Here's how the part is built. I have some questions about the finished solid (model axes, mm). Face numbers are marked on the shaded views. Give positions to 0.01 mm unless a question says otherwise; leave off trailing zeros. Order: outer loops, then holes, each group sorted by start corner. A loop starts at its lowest first (then second) coordinate and runs counter-clockwise, first axis right, second up. Notation, with made-up numbers: (49.25, 13) -> (63.25, 13) arc R20 cw to (63.25, 20) -> close; hole circle Ø2 at (35, 25.25). An arc over 180 degrees is marked (long way). Write each question's results on one line, items separated by ' | '. Start each with the question number.
Q1. I need wall thicknesses on line 1 along X through (y, z) = (0, 10.5); line 2 along X through (y, z) = (0, 24.5); line 3 along Z through (x, y) = (-1, 4). Which ranges of each line are inside material? Lowest first, please. Write a range as [from, to].
Q2. Thinking about a two-plate mould opening in Z: for the marked faces 1 and 2, which applies, pulls with the +Z half, pulls with the -Z half, needs draft (parallel to the pull), parting line crosses it, or undercut?
Q3. Imagine slicing it at C-C, the plane z = 27.75. Please give me the cut outline in (x, y).
Q4. I'm going to push a flat-ended pin straight in: pin 1 (1 mm diameter, centred on x = 3.5, y = 2, fed in from +Z). Where does the tip first touch, or does it pass through?
```python
from build123d import *

# Parameters (mm, degrees)
F0_R      = 5
F0_R_2    = 3.81
F1_DEPTH  = 28
F3_R      = 4.2
F4_DEPTH  = 10
F5_R      = 6.6272432787
F6_DEPTH  = 10
F2_R      = 4.2
F7_DEPTH  = 17
F9_DEPTH  = 6
F10_R     = 4.2
F11_DEPTH = 2
F12_R     = 5
F12_R_2   = 3
F13_DEPTH = 5
F14_R     = 1.99999


# Not quite as in the source:
# - a fillet or chamfer is up to 0.001 mm smaller than in the source, because OpenCascade refuses the exact size


with BuildPart() as f1:
    # F0 (on Top) → F1 (new body)
    with BuildSketch(Plane.XY):
        Circle(F0_R)
        Circle(F0_R_2, mode=Mode.SUBTRACT)
    extrude(amount=F1_DEPTH)

    # F3 (on face) → F4 (cut)
    with BuildSketch(Plane(origin=(0, 0, 0), x_dir=(1, 0, 0), z_dir=(0, 0, -1))):
        with Locations((0.1565692156, 0)):
            Circle(F3_R)
    extrude(amount=-F4_DEPTH, mode=Mode.SUBTRACT)

    # F5 (on face) → F6 (cut)
    with BuildSketch(Plane(origin=(0, 0, 0), x_dir=(1, 0, 0), z_dir=(0, 0, -1))):
        with Locations((-0.2925955923, 0)):
            Circle(F5_R)
    extrude(amount=-F6_DEPTH, mode=Mode.SUBTRACT)

    # F2 (on face) → F7 (cut)
    with BuildSketch(Plane.XY.offset(28)):
        Circle(F2_R)
    extrude(amount=-F7_DEPTH, mode=Mode.SUBTRACT)

    # F8 (on face) → F9 (join)
    with BuildSketch(Plane.XY.offset(28)):
        with BuildLine():
            ThreePointArc((1.8834823008, 3.7539971261), (0.2542086961, 4.2354191199), (-1.4209507588, 3.9523282937))
            ThreePointArc((-1.4209507588, 3.9523282937), (0.1766375517, 2.9429916253), (1.8834823008, 3.7539971261))
        make_face()
    extrude(amount=-F9_DEPTH)

    # F10 (on face) → F11 (cut)
    with BuildSketch(Plane.XY.offset(28)):
        Circle(F10_R)
    extrude(amount=-F11_DEPTH, mode=Mode.SUBTRACT)

    # F12 (on face) → F13 (join)
    with BuildSketch(Plane.XY.offset(28)):
        Circle(F12_R)
        Circle(F12_R_2, mode=Mode.SUBTRACT)
    extrude(amount=F13_DEPTH)

    # F14 (radius 2 in the source; OpenCascade refuses exactly that, so slightly less here)
    f14_edges = [f1.edges().sort_by_distance(p)[0] for p in [
        (-3, 0, 33),
    ]]
    fillet(f14_edges, radius=F14_R)


solid = f1.part
```
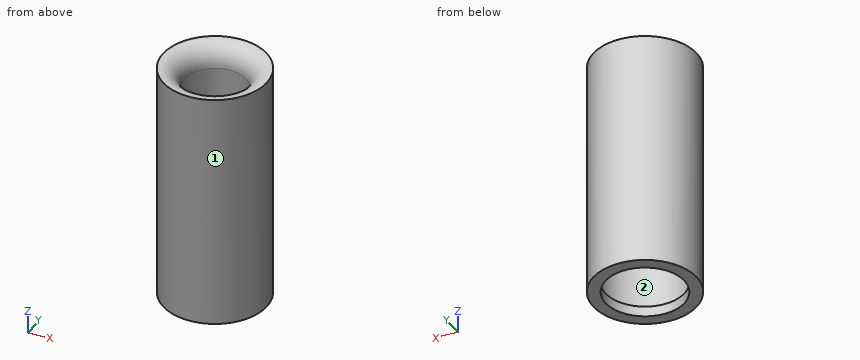
Geometry check:
1) line 1: [-5, -3.81], [3.81, 5] | line 2: [-5, -4.2], [4.2, 5] | line 3: [10, 11], [22, 26], [28, 32.8]
2) face 1: needs draft | face 2: undercut
3) outline: circle Ø10 at (0, 0); hole circle Ø8.4 at (0, 0)
4) pin 1: z = 32.94
